```python
from build123d import *
from build123d.topology import SkipClean

# Parameters (mm, degrees)
CROQUIS1_R              = 1.5
SALIENTE_EXTRUIR1_DEPTH = 15
CROQUIS2_R              = 2.5
CORTAR_EXTRUIR1_DEPTH   = 20
CORTAR_EXTRUIR2_DEPTH   = 22
CROQUIS4_W              = 3.68086323
CROQUIS4_H              = 12
CORTAR_EXTRUIR3_DEPTH   = 10
REDONDEO1_R             = 1.5


with BuildPart() as part:
    # Croquis1 → Saliente-Extruir1 (new body)
    with BuildSketch(Plane.XY):
        with BuildLine():
            Line((11.25, 14.1), (11.25, 11.1))
            Line((11.25, 11.1), (11.25, 5.1))
            Line((11.25, 5.1), (11.25, 2.1))
            Line((11.25, 2.1), (23.75, 2.1))
            Line((23.75, 2.1), (23.75, -0.9))
            Line((23.75, -0.9), (11.25, -0.9))
            Line((11.25, -0.9), (5.75, -0.9))
            ThreePointArc((5.75, -0.9), (0.800252532, 1.150252532), (-1.25, 6.1))
            Line((-1.25, 6.1), (-1.25, 10.1))
            ThreePointArc((-1.25, 10.1), (0.800252532, 15.049747468), (5.75, 17.1))
            Line((5.75, 17.1), (11.25, 17.1))
            Line((11.25, 17.1), (23.75, 17.1))
            Line((23.75, 17.1), (23.75, 14.1))
            Line((23.75, 14.1), (11.25, 14.1))
        make_face()
        with Locations((3.75, 8.1)):
            Circle(CROQUIS1_R, mode=Mode.SUBTRACT)
    extrude(amount=SALIENTE_EXTRUIR1_DEPTH)

    # Croquis2 → Cortar-Extruir1 (cut, symmetric)
    with BuildSketch(Plane(origin=(0, 0, 0), x_dir=(1, 0, 0), z_dir=(0, 1, 0))):
        with Locations(Location((17.5, -7.5, 0), (0, 0, 90))):
            Circle(CROQUIS2_R)
        with BuildLine():
            Line((17.5, -1.25), (11.25, 0))
            Line((11.25, 0), (11.126279301, 1.868603497))
            Line((11.126279301, 1.868603497), (29.663453957, 1.868603497))
            Line((29.663453957, 1.868603497), (29.663453957, -17.961269996))
            Line((29.663453957, -17.961269996), (11.25, -17.961269996))
            Line((11.25, -17.961269996), (11.25, -15))
            Line((11.25, -15), (17.5, -13.75))
            ThreePointArc((17.5, -13.75), (23.75, -7.5), (17.5, -1.25))
        make_face()
    extrude(amount=CORTAR_EXTRUIR1_DEPTH, both=True, mode=Mode.SUBTRACT)

    # Croquis3 → Cortar-Extruir2 (cut)
    with SkipClean():  # the faces are left unmerged after this step: merging them gives an invalid solid
        with BuildSketch(Plane(origin=(0, 17.1, 0), x_dir=(1, 0, 0), z_dir=(0, 1, 0))):
            Polygon((5.75, -10), (-2.050741432, -10), (-2.325121179, -18.2596058), (20.840368904, -18.2596058), (17.5, -13.75), (11.25, -15), (5.75, -15), align=None)
            with BuildLine():
                Line((9.25, -10), (5.75, -10))
                Line((5.75, -10), (5.75, -15))
                Line((5.75, -15), (11.25, -15))
                Line((11.25, -15), (17.5, -13.75))
                ThreePointArc((17.5, -13.75), (15.902831918, -13.542479137), (14.41172646, -12.933697318))
                Line((14.41172646, -12.933697318), (9.25, -10))
            make_face()
            with BuildLine():
                Line((5.75, 0), (5.75, -5))
                Line((5.75, -5), (9.25, -5))
                Line((9.25, -5), (14.41172646, -2.066302682))
                ThreePointArc((14.41172646, -2.066302682), (15.902831918, -1.457520863), (17.5, -1.25))
                Line((17.5, -1.25), (11.25, 0))
                Line((11.25, 0), (5.75, 0))
            make_face()
            Polygon((-2.050741432, -5), (5.75, -5), (5.75, 0), (11.25, 0), (17.5, -1.25), (17.5, 1.613327317), (-2.050741432, 1.613327317), align=None)
        extrude(amount=-CORTAR_EXTRUIR2_DEPTH, mode=Mode.SUBTRACT)

    # Croquis4 → Cortar-Extruir3 (cut, symmetric)
    with SkipClean():  # the faces are left unmerged after this step: merging them gives an invalid solid
        with BuildSketch(Plane.XY.offset(10)):
            with Locations((10.990431615, 8.1)):
                Rectangle(CROQUIS4_W, CROQUIS4_H)
        extrude(amount=CORTAR_EXTRUIR3_DEPTH, both=True, mode=Mode.SUBTRACT)

    # Redondeo1
    redondeo1_edges = [part.edges().sort_by_distance(p)[0] for p in [
        (9.15, 2.1, 7.5),
        (9.15, 14.1, 7.5),
    ]]
    fillet(redondeo1_edges, radius=REDONDEO1_R)


solid = part.part
```
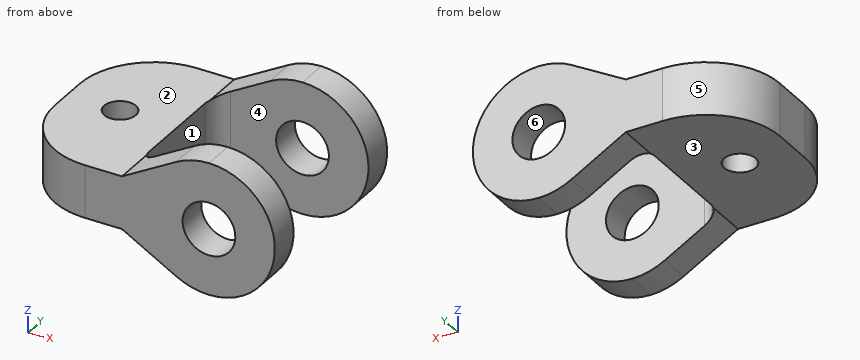
Verification items for the finished model (mm, model axes). Face numbers are marked on the shaded views. A direction names the side the tool comes from. Coordinates: 2 decimals unless noted, no trailing zeros. Order: outer loops, then holes, each group sorted by start corner. A loop starts at its lowest first (then second) coordinate and runs counter-clockwise, first axis right, second up. Notation, with made-up numbers: (28.25, 8.25) - (38.25, 8.25) arc R22 ccw to (38.25, 18.25) - close; hole circle Ø10 at (-30.5, -39). An arc over 180 degrees is marked (long way). Return JSON: item names as keys, results as strings.
(1) Section check A-A, the plane z = 7.5. Record the cut outline in (x, y), and give its area (3 significant figures).
Filled sheet:
{"outline": "(-1.25, 6.1) arc R7 ccw to (5.75, -0.9) - (15, -0.9) - (15, 2.1) - (10.65, 2.1) arc R1.5 cw to (9.15, 3.6) - (9.15, 12.6) arc R1.5 cw to (10.65, 14.1) - (15, 14.1) - (15, 17.1) - (5.75, 17.1) arc R7 ccw to (-1.25, 10.1) - close; (20, -0.9) - (23.75, -0.9) - (23.75, 2.1) - (20, 2.1) - close; (20, 14.1) - (23.75, 14.1) - (23.75, 17.1) - (20, 17.1) - close; hole circle Ø3 at (3.75, 8.1)", "area": "218 mm^2"}
(2) Section check D-D, the plane y = 0.5. Record the cut outline in (x, z).
Filled sheet:
{"outline": "(1.55, 5) - (9.25, 5) - (14.41, 2.07) arc R6.25 ccw (long way) to (14.41, 12.93) - (9.25, 10) - (1.55, 10) - close; hole circle Ø5 at (17.5, 7.5)"}
(3) Thickness scan on line 1 along Z through (x, y) = (17.5, 0.25); line 2 along Y through (x, z) = (17.75, 10.5); line 3 along X through (y, z) = (8.1, 6.95). Record the ranges inside material, lowest first.
Filled sheet:
{"line 1": "z = 1.25 to 5, 10 to 13.75", "line 2": "y = -0.9 to 2.1, 14.1 to 17.1", "line 3": "x = -1.25 to 2.25, 5.25 to 9.15"}
(4) Go/stop test with flat-tipped pins: pin 1 (5.5 mm diameter, centred on x = 3, y = 12, fed in from -Z); pin 2 (1 mm diameter, centred on y = 15, z = 8.5, fed in from +X); pin 3 (4 mm diameter, centred on y = 8.5, z = 9, fed in from +X). Record where each tip stops, or that it passes through.
Filled sheet:
{"pin 1": "stops at z = 5", "pin 2": "stops at x = 23.73", "pin 3": "stops at x = 9.15"}
(5) Section check C-C, the plane x = 16.25. Record the cut outline in (y, z).
Filled sheet:
{"outline": "(-0.9, 1.38) - (2.1, 1.38) - (2.1, 5.33) - (-0.9, 5.33) - close; (-0.9, 9.67) - (2.1, 9.67) - (2.1, 13.62) - (-0.9, 13.62) - close; (14.1, 1.38) - (17.1, 1.38) - (17.1, 5.33) - (14.1, 5.33) - close; (14.1, 9.67) - (17.1, 9.67) - (17.1, 13.62) - (14.1, 13.62) - close"}
(6) Mould release check, pull along Y, two halves, no side actions. Record for the marked faces 4, 5 and 6: pulls with the +Y half, pulls with the -Y half, needs draft (parallel to the pull), parting line crosses it, or undercut.
Filled sheet:
{"face 4": "undercut", "face 5": "pulls with the +Y half", "face 6": "needs draft"}
(7) Section check B-B, the plane y = 7.5. Record the cut outline in (x, z), and give its area (3 significant figures).
Filled sheet:
{"outline": "(-1.25, 5) - (2.38, 5) - (2.38, 10) - (-1.25, 10) - close; (5.12, 5) - (9.15, 5) - (9.15, 10) - (5.12, 10) - close", "area": "38.3 mm^2"}
(8) Access from +Z, -Z, +X, -X, +Y, -Y to the whole of each face (thin tool, end or side, straight path). Record for the marked faces 1, 2 and 3.
Filled sheet:
{"face 1": "+Z, -Z, +X", "face 2": "+Z, -X, +Y, -Y", "face 3": "-Z, -X, +Y, -Y"}
